Work out the finished part from the listing and answer in its coordinate system (mm). A direction names the side the tool comes from. Coordinates: 2 decimals unless noted, no trailing zeros. Loops run counter-clockwise (first coordinate to the right, second up) from the corner with the lowest first, then second, coordinate; pieces in that order, holes last. Notation, with made-up numbers: (68.25, 31) -> (96.25, 31) arc R23 cw to (96.25, 51) -> close; hole circle Ø5 at (79, 28.5). An arc over 180 degrees is marked (long way). Use a Markdown table: item, result. Add a question column.
Autodesk Inventor part; units mm, degrees
ref_plane "YZ Plane" through (0, 0, 0) normal (1, 0, 0) x (0, 1, 0)
ref_plane "XZ Plane" through (0, 0, 0) normal (0, 1, 0) x (-1, 0, 0)
ref_plane "XY Plane" through (0, 0, 0) normal (0, 0, 1) x (1, 0, 0)
sketch "Sketch4" plane through (0, 0, 0) normal (0, 1, 0) x (-1, 0, 0)
  line L0 (0, 0) -> (22.5, 0)
  line L1 (22.5, 0) -> (22.5, -77.5)
  line L2 (22.5, -77.5) -> (0, -77.5)
  line L3 (0, -77.5) -> (0, 0)
  arc A0 (0, -77.5) -> (22.5, -77.5) centre (11.25, -77.5) ccw
  arc A1 (22.5, 0) -> (0, 0) centre (11.25, 0) ccw
  dimension "d13" = 22.5
  dimension "d14" = 77.5
extrude "Extrusion10" add sketch "Sketch4" along normal blind 3 contours A1 L0 | L2 A0
sketch "Sketch13" plane through (0, 0, 0) normal (0, -1, 0) x (1, 0, 0)
  line L0 (0, 0) -> (-22.5, 0)
  line L1 (-22.5, -77.5) -> (0, -77.5)
  line L2 (0, 0) -> (-22.5, 0)
  line L3 (-22.5, 0) -> (-22.5, -77.5)
  line L4 (-22.5, -77.5) -> (0, -77.5)
  line L5 (0, -77.5) -> (0, 0)
extrude "Extrusion11" add sketch "Sketch13" against normal blind 3
sketch "Sketch17" plane through (0, 3, 0) normal (0, 1, 0) x (1, 0, 0)
  line L0 (-22.5, 77.5) -> (-22.5, 0)
  line L1 (-22.5, 0) -> (-21, 0)
  line L2 (-21, 0) -> (-21, 77.5)
  line L3 (-21, 77.5) -> (-22.5, 77.5)
  line L4 (-22.5, 77.5) -> (-22.5, 0)
  point P0 (0, 0)
  dimension "d82" = 1.5
extrude "Extrusion14" add sketch "Sketch17" along normal blind 9
sketch "Sketch18" plane through (0, 3, 0) normal (0, 1, 0) x (1, 0, 0)
  line L0 (0, 0) -> (0, 77.5)
  line L1 (-21, 0) -> (-21, 77.5)
  line L2 (0, 0) -> (-21, 0)
  line L3 (-21, 0) -> (-21, 1)
  line L4 (-21, 1) -> (0, 1)
  line L5 (0, 1) -> (0, 0)
  arc A0 (0, 77.5) -> (-22.5, 77.5) centre (-11.25, 77.5) ccw
  line L6 (0, 77.5) -> (-21, 77.5)
  line L7 (-21, 77.5) -> (-21, 76.5)
  line L8 (-21, 76.5) -> (0, 76.5)
  line L9 (0, 76.5) -> (0, 77.5)
  line L10 (-21, 37.5) -> (0, 37.5)
  line L11 (0, 37.5) -> (0, 40)
  line L12 (0, 40) -> (-21, 40)
  line L13 (-21, 40) -> (-21, 37.5)
  dimension "d85" = 1
  dimension "d86" = 1
  dimension "d87" = 2.5
  dimension "d88" = 36.5
extrude "Extrusion15" add sketch "Sketch18" along normal blind 9 contours L2 L1 L4 L0 | L10 L1 L12 L0 | L8 L1 L6 L0
sketch "Sketch19" plane through (0, 3, 0) normal (0, 1, 0) x (1, 0, 0)
  line L0 (0, 77.5) -> (-22.5, 77.5)
  circle A0 centre (-11.25, 83.125) radius 1.75
  arc A1 (-22.5, 0) -> (0, 0) centre (-11.25, 0) ccw
  circle A2 centre (-11.25, -5.625) radius 1.75
  dimension "d92" = 3.5
  dimension "d94" = 3.5
hole "Hole3" at (-11.25, 3, -83.125) at (-11.25, 3, 5.625) direction (0, -1, 0) diameter 3.5 end through all
properties part number "Wago Terminal Block New"
Item 1: Find the intervals of material crossed by probe 1 along Z at (x, y) = (-20.25, 4.75); probe 2 along Z at (x, y) = (-11.25, 2.25) (3 decimals); probe 3 along X at (y, z) = (6, -62), in increasing order.
Item 2: Section A-A (x = -11.25) is taken. Determine the outline of the cut face in (y, z) (3 decimals).
Item 3: Section C-C (z = 5.5) is taken. Determine the outline of the cut face in (x, y).
Item 4: Given pin 1 (6.5 mm diameter, centred on x = -7, z = -21.5, fed in from +Y); pin 2 (1 mm diameter, centred on y = 8, z = -6, fed in from +X); pin 3 (7 mm diameter, centred on x = -9, y = 6, fed in from +Z), each flat-ended and moving along its own axis, determine where each tip first touches the part or whether it passes through.
Item 5: For faces 4 (the face through (-11, 7, 0)), 5 (the face through (-11, 7, -76.5)), 6 (the face through (-11, 3, -81)), 7 (the face through (-22.5, 6, -39)), determine the directions among +Z, -Z, +X, -X, +Y, -Y from which every point of the face is accessible in a straight line to the end or side of a thin tool.
Item 6: For a pull along X with two mould halves and no side action, classify faces 1 (the face through (-11, 7, -77.5)), 2 (the face through (-12.985, 1.479, 5.397)), 3 (the face through (-21, 7, -19)) as +X half, -X half, draft (parallel to the pull), parting line (faces both ways), or undercut.
Item 7: Section B-B (y = 6.5) is taken. Determine the outline of the cut face in (x, z).
Item 8: Section D-D (z = -28) is taken. Determine the outline of the cut face in (x, y).
Output:
| question | item | result |
|---|---|---|
| 1 | probe 1 | z = -77.5 to -76.5, -40 to -37.5, -1 to 0 |
| 1 | probe 2 | z = -88.75 to -84.875, -81.375 to 3.875, 7.375 to 11.25 |
| 1 | probe 3 | x = -22.5 to -21 |
| 2 | outline | (0, -88.75) -> (3, -88.75) -> (3, -84.875) -> (0, -84.875) -> close; (0, -81.375) -> (3, -81.375) -> (3, -77.5) -> (12, -77.5) -> (12, -76.5) -> (3, -76.5) -> (3, -40) -> (12, -40) -> (12, -37.5) -> (3, -37.5) -> (3, -1) -> (12, -1) -> (12, 0) -> (3, 0) -> (3, 3.875) -> (0, 3.875) -> close; (0, 7.375) -> (3, 7.375) -> (3, 11.25) -> (0, 11.25) -> close |
| 3 | outline | (-21.06, 0) -> (-13, 0) -> (-13, 3) -> (-21.06, 3) -> close; (-9.5, 0) -> (-1.44, 0) -> (-1.44, 3) -> (-9.5, 3) -> close |
| 4 | pin 1 | stops at y = 3 |
| 4 | pin 2 | stops at x = -21 |
| 4 | pin 3 | stops at z = 11.24 |
| 5 | face 4 | +Z, +X, -X, +Y |
| 5 | face 5 | +X, +Y |
| 5 | face 6 | -Z, +X, -X, +Y |
| 5 | face 7 | +Z, -Z, -X, +Y, -Y |
| 6 | face 1 | draft |
| 6 | face 2 | undercut |
| 6 | face 3 | +X half |
| 7 | outline | (-22.5, -77.5) -> (0, -77.5) -> (0, -76.5) -> (-21, -76.5) -> (-21, -40) -> (0, -40) -> (0, -37.5) -> (-21, -37.5) -> (-21, -1) -> (0, -1) -> (0, 0) -> (-22.5, 0) -> close |
| 8 | outline | (-22.5, 0) -> (0, 0) -> (0, 3) -> (-21, 3) -> (-21, 12) -> (-22.5, 12) -> close |
